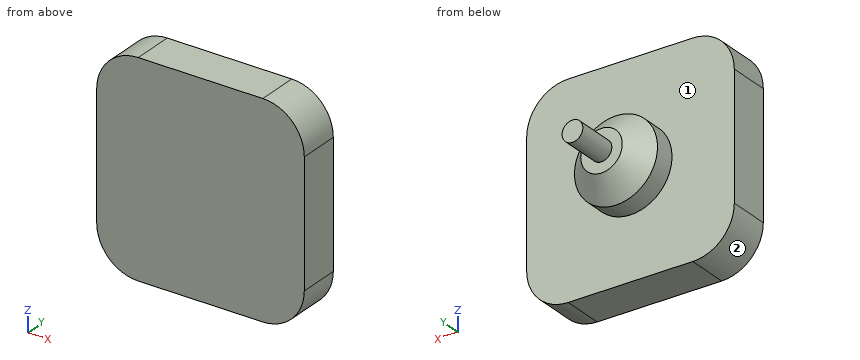
from build123d import *

# Parameters (mm, degrees)
SKETCH1_W           = 500
SKETCH1_H           = 500
BOSS_EXTRUDE1_DEPTH = 100
SKETCH2_R           = 100
BOSS_EXTRUDE2_DEPTH = 100
SKETCH3_R           = 25
BOSS_EXTRUDE3_DEPTH = 100
CHAMFER1_SIZE       = 50
FILLET1_R           = 100


with BuildPart() as part:
    # Sketch1 → Boss-Extrude1 (new body)
    with BuildSketch(Plane(origin=(0, 0, 0), x_dir=(1, 0, 0), z_dir=(0, 1, 0))):
        Rectangle(SKETCH1_W, SKETCH1_H)
    extrude(amount=BOSS_EXTRUDE1_DEPTH)

    # Sketch2 → Boss-Extrude2 (add)
    with BuildSketch(Plane(origin=(0, 100, 0), x_dir=(1, 0, 0), z_dir=(0, 1, 0))):
        Circle(SKETCH2_R)
    extrude(amount=BOSS_EXTRUDE2_DEPTH)

    # Sketch3 → Boss-Extrude3 (add)
    with BuildSketch(Plane(origin=(0, 200, 0), x_dir=(1, 0, 0), z_dir=(0, 1, 0))):
        Circle(SKETCH3_R)
    extrude(amount=BOSS_EXTRUDE3_DEPTH)

    # Chamfer1
    chamfer1_edges = [part.edges().sort_by_distance(p)[0] for p in [
        (-100, 200, 0),
    ]]
    chamfer(chamfer1_edges, length=CHAMFER1_SIZE)

    # Fillet1
    fillet1_edges = [part.edges().sort_by_distance(p)[0] for p in [
        (250, 50, 250),
        (-250, 50, 250),
        (-250, 50, -250),
        (250, 50, -250),
    ]]
    fillet(fillet1_edges, radius=FILLET1_R)


solid = part.part
Can you work these out from the model? Positions are in its coordinate system, mm. Face numbers are marked on the shaded views. A direction names the side the tool comes from. Round coordinates to 2 decimals unless told otherwise and drop trailing zeros. Write each loop counter-clockwise with the first axis right and the second up, starting at its lowest first coordinate (ties: lowest second). Pieces come first, ordered by that corner, then holes. Notation, with made-up numbers: (20, -35) - (65, -35) arc R10 cw to (65, -20) - close; hole circle Ø8 at (-30.75, 7.25). An arc over 180 degrees is marked (long way). Write each question's results on one line, items separated by ' | '. Start each with the question number.
1) Which directions (+Z, -Z, +X, -X, +Y, -Y) give clear straight access to the entire face, cutting with the end or side of a thin tool? Please do the marked faces 1 and 2.
2) Please list where these lines run through material, in increasing order: line 1 (Y direction, x = 76, z = -215.5); line 2 (Z direction, x = -155, y = 30); line 3 (X direction, y = 95.5, z = -154.5).
3) Suppose I cut it at D-D (x = 136). List the corners of the cut face in (y, z) for me.
4) Suppose I cut it at B-B (y = 85). List the corners of the cut face in (x, z) for me.
5) Suppose I cut it at C-C (z = 0). List the corners of the cut face in (x, y) for me.
6) For pin 1 Ø5 at (x, z) = (-168, 191.5) entering from +Y; pin 2 Ø1 at (y, z) = (104.5, -20) entering from +X, each with a flat end and sliding along its axis, tell me the tip position at first contact or that it passes through.
7) Suppose I cut it at A-A (x = 0). List the corners of the cut face in (y, z) for me, and give its area (3 significant figures).
Here are the results:
1) face 1: +Y | face 2: -Z, -X, +Y, -Y
2) line 1: y = 0 to 100 | line 2: z = -249.87 to 249.87 | line 3: x = -249.9 to 249.9
3) outline: (0, -250) - (100, -250) - (100, 250) - (0, 250) - close
4) outline: (-250, -150) arc R100 ccw to (-150, -250) - (150, -250) arc R100 ccw to (250, -150) - (250, 150) arc R100 ccw to (150, 250) - (-150, 250) arc R100 ccw to (-250, 150) - close
5) outline: (-250, 0) - (250, 0) - (250, 100) - (100, 100) - (100, 150) - (50, 200) - (25, 200) - (25, 300) - (-25, 300) - (-25, 200) - (-50, 200) - (-100, 150) - (-100, 100) - (-250, 100) - close
6) pin 1: stops at y = 100 | pin 2: stops at x = 98.08
7) outline: (0, -250) - (100, -250) - (100, -100) - (150, -100) - (200, -50) - (200, -25) - (300, -25) - (300, 25) - (200, 25) - (200, 50) - (150, 100) - (100, 100) - (100, 250) - (0, 250) - close | area: 72,500 mm2
